Work out the finished part from the listing and answer in its coordinate system (mm). Face numbers are marked on the shaded views. A direction names the side the tool comes from. Round coordinates to 2 decimals unless told otherwise and drop trailing zeros. Write each loop counter-clockwise with the first axis right and the second up, starting at its lowest first coordinate (ties: lowest second). Pieces come first, ordered by that corner, then holes. Notation, with made-up numbers: M 36.5,-31 L 92.5,-31 A18 ccw 92.5,-5 Z; hole C -5.5,23 d6. An arc over 180 degrees is marked long. Answer in a Markdown table with one row per item.
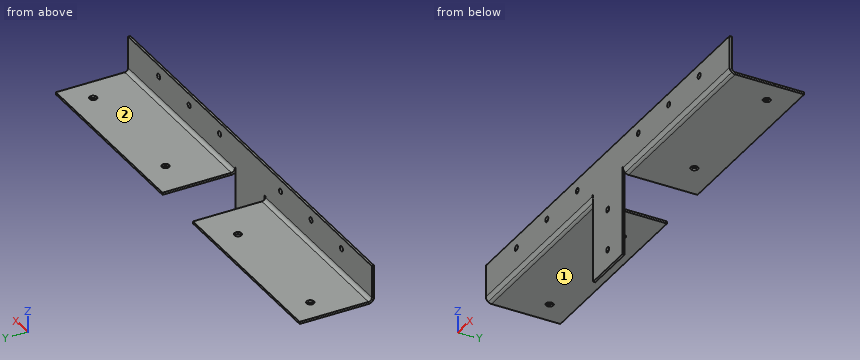
```python
from build123d import *

# Parameters (mm, degrees)
SKETCH1_W                    = 406.4
SKETCH1_H                    = 111.125
BASE_FLANGE1_DEPTH           = 2.032
EDGE_FLANGE2_START           = -203.2
EDGE_FLANGE2_DEPTH           = 178.816
EDGE_FLANGE2_START_2         = -25.4
EDGE_FLANGE2_2_DEPTH         = 1.016
EDGE_FLANGE2_3_DEPTH         = 177.8
EDGE_FLANGE3_START           = 24.384
EDGE_FLANGE3_DEPTH           = 178.816
EDGE_FLANGE3_2_DEPTH         = 1.016
EDGE_FLANGE3_START_2         = 25.4
EDGE_FLANGE3_3_DEPTH         = 177.8
SKETCH24_W                   = 177.8
SKETCH24_H                   = 2.032
BOSS_EXTRUDE1_DEPTH          = 5.4229
F_10_0_1935_DIAMETER_HOLE1_D = 4.9149
F_1_4_CLEARANCE_HOLE1_D      = 6.7564


# Read off the part's stored shape, not the designer's step: Edge-Flange2, Edge-Flange3
# Sheet-metal steps are written as plain solids
with BuildPart() as part:
    # Sketch1 → Base-Flange1 (new body)
    with BuildSketch(Plane(origin=(0, 0, 0), x_dir=(1, 0, 0), z_dir=(0, 1, 0))):
        with Locations((0, 55.5625)):
            Rectangle(SKETCH1_W, SKETCH1_H)
    extrude(amount=-BASE_FLANGE1_DEPTH)

    # Edge-Flange2 outline → Edge-Flange2 (cut)
    with BuildSketch(Plane.YZ.offset(EDGE_FLANGE2_START)):
        with BuildLine():
            ThreePointArc((0, -33.84501151), (-1.496459836, -32.018067825), (-2.032, -29.718))
            Line((-2.032, -29.718), (-2.032, -111.125))
            Line((-2.032, -111.125), (0, -111.125))
            Line((0, -111.125), (0, -33.84501151))
        make_face()
    extrude(amount=EDGE_FLANGE2_DEPTH, mode=Mode.SUBTRACT)

    # Edge-Flange2 2 outline → Edge-Flange2 2 (cut)
    with BuildSketch(Plane.YZ.offset(EDGE_FLANGE2_START_2)):
        with BuildLine():
            Line((0, -28.702), (-2.032, -28.702))
            Line((-2.032, -28.702), (-2.032, -29.718))
            ThreePointArc((-2.032, -29.718), (-1.496459836, -32.018067825), (0, -33.84501151))
            Line((0, -33.84501151), (0, -28.702))
        make_face()
    extrude(amount=EDGE_FLANGE2_2_DEPTH, mode=Mode.SUBTRACT)

    # Edge-Flange2 3 outline → Edge-Flange2 3 (add)
    with BuildSketch(Plane.YZ.offset(EDGE_FLANGE2_START)):
        with BuildLine():
            ThreePointArc((3.175, -32.893), (0.92993597, -31.96306403), (0, -29.718))
            Line((0, -29.718), (0, -33.84501151))
            ThreePointArc((0, -33.84501151), (1.498172628, -34.647614485), (3.175, -34.925))
            Line((3.175, -34.925), (61.468, -34.925))
            Line((61.468, -34.925), (61.468, -32.893))
            Line((61.468, -32.893), (3.175, -32.893))
        make_face()
    extrude(amount=EDGE_FLANGE2_3_DEPTH)

    # Edge-Flange3 outline → Edge-Flange3 (cut)
    with BuildSketch(Plane.YZ.offset(EDGE_FLANGE3_START)):
        with BuildLine():
            ThreePointArc((0, -33.84501151), (-1.496459836, -32.018067825), (-2.032, -29.718))
            Line((-2.032, -29.718), (-2.032, -111.125))
            Line((-2.032, -111.125), (0, -111.125))
            Line((0, -111.125), (0, -33.84501151))
        make_face()
    extrude(amount=EDGE_FLANGE3_DEPTH, mode=Mode.SUBTRACT)

    # Edge-Flange3 2 outline → Edge-Flange3 2 (cut)
    with BuildSketch(Plane.YZ.offset(EDGE_FLANGE3_START)):
        with BuildLine():
            Line((0, -28.702), (-2.032, -28.702))
            Line((-2.032, -28.702), (-2.032, -29.718))
            ThreePointArc((-2.032, -29.718), (-1.496459836, -32.018067825), (0, -33.84501151))
            Line((0, -33.84501151), (0, -28.702))
        make_face()
    extrude(amount=EDGE_FLANGE3_2_DEPTH, mode=Mode.SUBTRACT)

    # Edge-Flange3 3 outline → Edge-Flange3 3 (add)
    with BuildSketch(Plane.YZ.offset(EDGE_FLANGE3_START_2)):
        with BuildLine():
            ThreePointArc((3.175, -32.893), (0.92993597, -31.96306403), (0, -29.718))
            Line((0, -29.718), (0, -33.84501151))
            ThreePointArc((0, -33.84501151), (1.498172628, -34.647614485), (3.175, -34.925))
            Line((3.175, -34.925), (61.468, -34.925))
            Line((61.468, -34.925), (61.468, -32.893))
            Line((61.468, -32.893), (3.175, -32.893))
        make_face()
    extrude(amount=EDGE_FLANGE3_3_DEPTH)

    # Sketch24 → Boss-Extrude1 (add)
    with BuildSketch(Plane(origin=(0, 61.468, 0), x_dir=(1, 0, 0), z_dir=(0, 1, 0))):
        with Locations((-114.3, 33.909)):
            Rectangle(SKETCH24_W, SKETCH24_H)
        with Locations((114.3, 33.909)):
            Rectangle(SKETCH24_W, SKETCH24_H)
    extrude(amount=BOSS_EXTRUDE1_DEPTH)

    # #10 (0.1935) Diameter Hole1 (through all)
    with Locations(Plane(origin=(0, 0, 0), x_dir=(1, 0, 0), z_dir=(0, 1, 0))):
        with Locations((0, 93.853), (0, 55.753), (-152.4, 10.6172), (-50.8, 10.6172), (152.4, 10.6172), (50.8, 10.6172), (101.6, 10.6172), (-101.6, 10.6172)):
            Hole(F_10_0_1935_DIAMETER_HOLE1_D / 2)

    # 1/4 Clearance Hole1 (through all)
    with Locations(Plane(origin=(0, 0, -34.925), x_dir=(-1, 0, 0), z_dir=(0, 0, -1))):
        with Locations((180.975, 44.6659), (60.325, 44.6659), (-180.975, 44.6659), (-60.325, 44.6659)):
            Hole(F_1_4_CLEARANCE_HOLE1_D / 2)


solid = part.part
```
1. The part is cut by section C-C (z = -68). Determine the outline of the cut face in (x, y), plus the area to 3 significant figures.
Calculated:
| item | result |
|---|---|
| outline | M -24.38,-2.03 L 24.38,-2.03 L 24.38,0 L -24.38,0 Z |
| area | 99.1 mm² |
2. The part is cut by section A-A (y = 29.5). Determine the outline of the cut face in (x, z) (3 decimals).
Calculated:
| item | result |
|---|---|
| outline | M -203.2,-34.925 L -25.4,-34.925 L -25.4,-32.893 L -203.2,-32.893 Z; M 25.4,-34.925 L 203.2,-34.925 L 203.2,-32.893 L 25.4,-32.893 Z |
3. Given pin 1 (9 mm diameter, centred on x = -180.98, y = 44.67, fed in from -Z) (3 decimals); pin 2 (3 mm diameter, centred on y = 23, z = -31.5, fed in from +X); pin 3 (5.5 mm diameter, centred on x = -101.6, z = -10.62, fed in from +Y); pin 4 (3 mm diameter, centred on x = -104, y = 11, fed in from +Z), each flat-ended and moving along its own axis, determine where each tip first touches the part or whether it passes through.
Calculated:
| item | result |
|---|---|
| pin 1 | stops at z = -34.925 |
| pin 2 | stops at x = 203.2 |
| pin 3 | stops at y = 0 |
| pin 4 | stops at z = -32.89 |
4. Consider line 1 along Z through (x, y) = (186, 18.5) (3 decimals); line 2 along Y through (x, z) = (4, -56.5); line 3 along Z through (x, y) = (50.8, -1.1). Determine where each line is inside the solid, lowest interval first. Write a range as from..to.
Calculated:
| item | result |
|---|---|
| line 1 | z = -34.925..-32.893 |
| line 2 | y = -2.03..0 |
| line 3 | z = -32.69..-13.07, -8.16..0 |
5. A tool of negligible diameter and unlimited length cuts with its end or side. For the marked faces 1 and 2, from which of +Z, -Z, +X, -X, +Y, -Y can it reach the whole face along a straight path? Write none if from no direction.
Calculated:
| item | result |
|---|---|
| face 1 | -Z, +X, -X, +Y, -Y |
| face 2 | +Z, +X, -X, +Y |
6. The part is cut by section B-B (x = 165). Determine the outline of the cut face in (y, z) (3 decimals).
Calculated:
| item | result |
|---|---|
| outline | M -2.032,-29.718 A5.207 ccw 3.175,-34.925 L 66.891,-34.925 L 66.891,-32.893 L 3.175,-32.893 A3.175 cw 0,-29.718 L 0,0 L -2.032,0 Z |
7. The part is cut by section D-D (x = 20). Determine the outline of the cut face in (y, z) (3 decimals).
Calculated:
| item | result |
|---|---|
| outline | M -2.032,-111.125 L 0,-111.125 L 0,0 L -2.032,0 Z |
